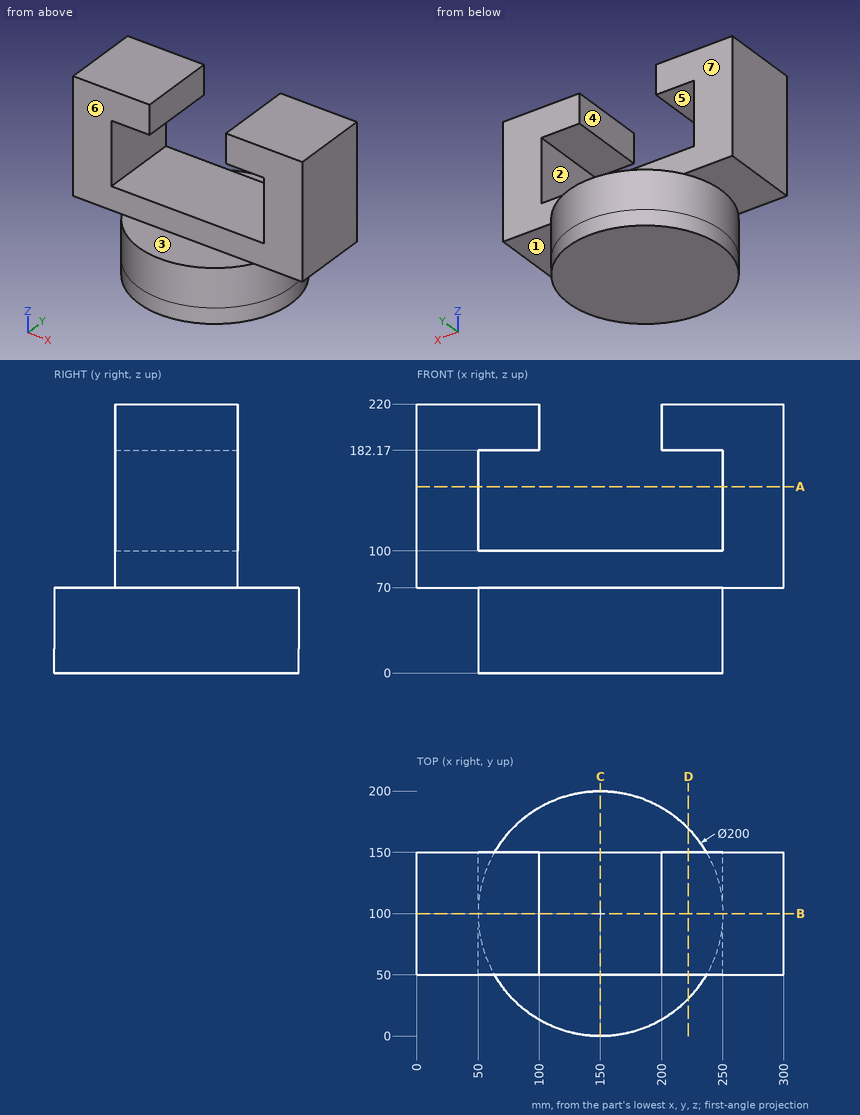
Geometry check sheet. Reference: drawing and pictorial views, mm from the part's lowest x, y, z. A direction names the side the tool comes from. Round coordinates to 2 decimals unless told otherwise and drop trailing zeros. Order: outer loops, then holes, each group sorted by start corner. A loop starts at its lowest first (then second) coordinate and runs counter-clockwise, first axis right, second up. Notation, with made-up numbers: M 16,87 L 45,87 A30 cw 45,112 Z; hole C -11,-32 d11. An arc over 180 degrees is marked long. Answer in a Markdown table with one row per item.
(1) Go/stop test with flat-tipped pins: P1, Ø2, axis at x = 180, y = 57.5, coming from the -Z side; P2, Ø6, axis at y = 50, z = 57.5, coming from the -X side; P3, Ø1.5, axis at x = 184.5, y = 128.5, coming from the +Z side; P4, Ø19, axis at x = 18, y = 111, coming from the -Z side. Record where each tip stops, or that it passes through.
Responses:
| item | result |
|---|---|
| P1 | stops at z = 0 |
| P2 | stops at x = 61.73 |
| P3 | stops at z = 100 |
| P4 | stops at z = 70 |
(2) Tool access check on the marked faces 4, 5, 6 and 7. Record the directions out of +Z, -Z, +X, -X, +Y, -Y that give a thin tool (end or side, any length) a straight path to the whole face; none if there is none.
Responses:
| item | result |
|---|---|
| face 4 | +Z, +Y, -Y |
| face 5 | +Y, -Y |
| face 6 | +Z, +X, -X, -Y |
| face 7 | +Z, +X, -X, +Y |
(3) Sectioned sample at B-B, the plane y = 100. Record the cut outline in (x, z), and give its area (3 significant figures).
Responses:
| item | result |
|---|---|
| outline | M 0,70 L 50,70 L 50,0 L 250,0 L 250,70 L 300,70 L 300,220 L 200,220 L 200,182.17 L 250,182.17 L 250,100 L 50,100 L 50,182.17 L 100,182.17 L 100,220 L 0,220 Z |
| area | 38,800 mm² |
(4) Draft check along Z on the marked faces 1, 2 and 3. Enter one of: released by +Z, released by -Z, zero draft, split by the parting line, or undercut.
Responses:
| item | result |
|---|---|
| face 1 | released by -Z |
| face 2 | undercut |
| face 3 | released by +Z |
(5) Sectioned sample at D-D, the plane x = 222. Record the cut outline in (y, z), and give its area (3 significant figures).
Responses:
| item | result |
|---|---|
| outline | M 30.6,0 L 169.4,0 L 169.4,70 L 150,70 L 150,100 L 50,100 L 50,70 L 30.6,70 Z; M 50,182.17 L 150,182.17 L 150,220 L 50,220 Z |
| area | 16,500 mm² |
(6) Sectioned sample at A-A, the plane z = 152.5. Record the cut outline in (x, y), and give its area (3 significant figures).
Responses:
| item | result |
|---|---|
| outline | M 0,50 L 50,50 L 50,150 L 0,150 Z; M 250,50 L 300,50 L 300,150 L 250,150 Z |
| area | 10,000 mm² |
(7) Sectioned sample at C-C, the plane x = 150. Record the cut outline in (y, z).
Responses:
| item | result |
|---|---|
| outline | M 0,0 L 200,0 L 200,70 L 150,70 L 150,100 L 50,100 L 50,70 L 0,70 Z |
(8) Scan lines: probe 1 along X at (y, z) = (111, 113); probe 2 along Z at (x, y) = (86, 100.5); probe 3 along Y at (x, z) = (181, 98). Record each from-to range of solid material in increasing order. Write a range as from..to.
Responses:
| item | result |
|---|---|
| probe 1 | x = 0..50, 250..300 |
| probe 2 | z = 0..100, 182.17..220 |
| probe 3 | y = 50..150 |
